Model file for the job. Use its own axes, mm. Give positions to 0.01 mm unless a question says otherwise; leave off trailing zeros. Loops run counter-clockwise (first coordinate to the right, second up) from the corner with the lowest first, then second, coordinate; pieces in that order, holes last. Notation, with made-up numbers: M 14,9.5 L 22,9.5 A15 cw 22,23.5 Z; hole C -6.75,11.5 d11. An arc over 180 degrees is marked long. Answer in a Markdown table with one row per item.
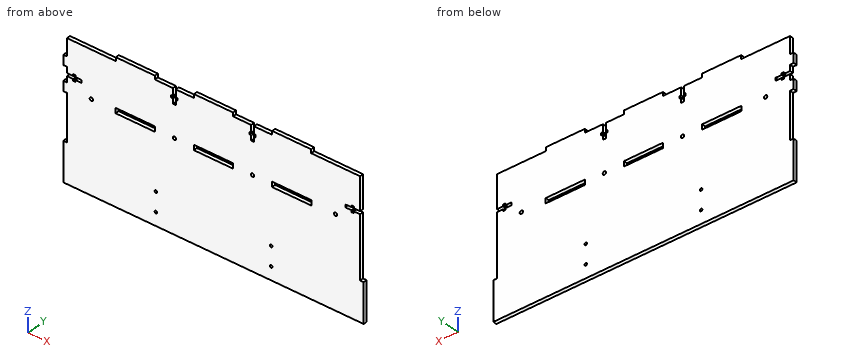
```python
from build123d import *

# Parameters (mm, degrees)
F0_R     = 1.5875
F0_W     = 51.054
F0_H     = 6.604
F0_W_2   = 4.7625
F0_H_2   = 50.8
F0_W_3   = 50.8
F0_H_3   = 4.7625
F0_H_4   = 12.7
F1_DEPTH = 4.7625
F2_D     = 4.318
F2_DEPTH = 11.9126
F2_TIP   = 1.2972580765


with BuildPart() as f1:
    # F0 (on Front) → F1 (new body)
    with BuildSketch(Plane.XZ):
        Polygon((-127, 88.9), (-190.5, 88.9), (-190.5, 66.675), (-190.5, 53.975), (-190.5, 46.2915), (-182.5625, 46.2915), (-182.5625, 48.5775), (-179.3875, 48.5775), (-179.3875, 46.2915), (-171.45, 46.2915), (-171.45, 42.6085), (-179.3875, 42.6085), (-179.3875, 40.3225), (-182.5625, 40.3225), (-182.5625, 42.6085), (-190.5, 42.6085), (-190.5, 34.925), (-190.5, 22.225), (-190.5, -38.1), (-190.5, -88.9), (190.5, -88.9), (190.5, -38.1), (190.5, 22.225), (190.5, 34.925), (190.5, 42.6085), (182.5625, 42.6085), (182.5625, 40.3225), (179.3875, 40.3225), (179.3875, 42.6085), (171.45, 42.6085), (171.45, 46.2915), (179.3875, 46.2915), (179.3875, 48.5775), (182.5625, 48.5775), (182.5625, 46.2915), (190.5, 46.2915), (190.5, 53.975), (190.5, 66.675), (190.5, 88.9), (127, 88.9), (76.2, 88.9), (52.6415, 88.9), (52.6415, 79.375), (54.9275, 79.375), (54.9275, 76.2), (52.6415, 76.2), (52.6415, 69.85), (48.9585, 69.85), (48.9585, 76.2), (46.6725, 76.2), (46.6725, 79.375), (48.9585, 79.375), (48.9585, 88.9), (25.4, 88.9), (-25.4, 88.9), (-48.9585, 88.9), (-48.9585, 79.375), (-46.6725, 79.375), (-46.6725, 76.2), (-48.9585, 76.2), (-48.9585, 69.85), (-52.6415, 69.85), (-52.6415, 76.2), (-54.9275, 76.2), (-54.9275, 79.375), (-52.6415, 79.375), (-52.6415, 88.9), (-76.2, 88.9), align=None)
        with Locations((-74.9310097456, -71.9249998569)):
            Circle(F0_R, mode=Mode.SUBTRACT)
        with Locations((-74.9310097456, -46.9249998569)):
            Circle(F0_R, mode=Mode.SUBTRACT)
        with Locations((75.0689902544, -71.9249998569)):
            Circle(F0_R, mode=Mode.SUBTRACT)
        with Locations((75.0689902544, -46.9249998569)):
            Circle(F0_R, mode=Mode.SUBTRACT)
        with Locations((-101.6, 28.575)):
            Rectangle(F0_W, F0_H, mode=Mode.SUBTRACT)
        with Locations((0, 28.575)):
            Rectangle(F0_W, F0_H, mode=Mode.SUBTRACT)
        with Locations((101.6, 28.575)):
            Rectangle(F0_W, F0_H, mode=Mode.SUBTRACT)
        with Locations((192.88125, -63.5)):
            Rectangle(F0_W_2, F0_H_2)
        with Locations((-192.88125, -63.5)):
            Rectangle(F0_W_2, F0_H_2)
        with Locations((-101.6, 91.28125)):
            Rectangle(F0_W_3, F0_H_3)
        with Locations((0, 91.28125)):
            Rectangle(F0_W_3, F0_H_3)
        with Locations((101.6, 91.28125)):
            Rectangle(F0_W_3, F0_H_3)
        with Locations((-192.88125, 60.325)):
            Rectangle(F0_W_2, F0_H_4)
        with Locations((-192.88125, 28.575)):
            Rectangle(F0_W_2, F0_H_4)
    extrude(amount=F1_DEPTH)

    # F2
    with Locations(Plane(origin=(0, 0, 0), x_dir=(1, 0, 0), z_dir=(0, 1, 0))):
        with Locations((-158.75, -28.575), (-50.7365, -28.575), (50.8, -28.575), (158.75, -28.575)):
            Hole(F2_D / 2, depth=F2_DEPTH)
            with Locations((0, 0, -(F2_DEPTH + F2_TIP / 2))):  # 118° drill point
                Cone(0, F2_D / 2, F2_TIP, mode=Mode.SUBTRACT)


solid = f1.part
```
(1) Saw through at C-C, the plane z = -3. Give the cut face in (x, y), and give its area (3 significant figures).
Established:
| item | result |
|---|---|
| outline | M -190.5,-4.76 L 190.5,-4.76 L 190.5,0 L -190.5,0 Z |
| area | 1,810 mm2 |
(2) Saw through at A-A, the plane x = -13.5. Give the cut face in (y, z).
Established:
| item | result |
|---|---|
| outline | M -4.76,-88.9 L 0,-88.9 L 0,25.27 L -4.76,25.27 Z; M -4.76,31.88 L 0,31.88 L 0,93.66 L -4.76,93.66 Z |
(3) Saw through at D-D, the plane y = -1.9. Count the separate pieces of the cut face and the enclosed holes in it, and give its area (3 significant figures).
Established:
| item | result |
|---|---|
| separate pieces | 1 |
| enclosed holes | 11 |
| area | 67,600 mm2 |
(4) Flat gauge pins, fed straight in: P1, Ø12, axis at x = -112, z = -67, coming from the +Y side; P2, Ø1, axis at x = -139, y = -2, coming from the +Z side; P3, Ø1.5, axis at y = -1.5, z = 73, coming from the -X side. Where does each tip first touch, or does it go through?
Established:
| item | result |
|---|---|
| P1 | stops at y = 0 |
| P2 | stops at z = 88.9 |
| P3 | stops at x = -190.5 |
(5) Saw through at B-B, the plane x = 143.5. Give the cut face in (y, z), and give its area (3 significant figures).
Established:
| item | result |
|---|---|
| outline | M -4.76,-88.9 L 0,-88.9 L 0,88.9 L -4.76,88.9 Z |
| area | 847 mm2 |
(6) Wall check: L1, parallel to X at y = -2.9, z = 80; L2, parallel to X at y = -4.35, z = 41.5; L3, parallel to Z at x = 24, y = -2.3. Give the ranges that are in metal, low to high.
Established:
| item | result |
|---|---|
| L1 | x = -190.5 to -52.64, -48.96 to 48.96, 52.64 to 190.5 |
| L2 | x = -190.5 to -182.56, -179.39 to 179.39, 182.56 to 190.5 |
| L3 | z = -88.9 to 25.27, 31.88 to 93.66 |
